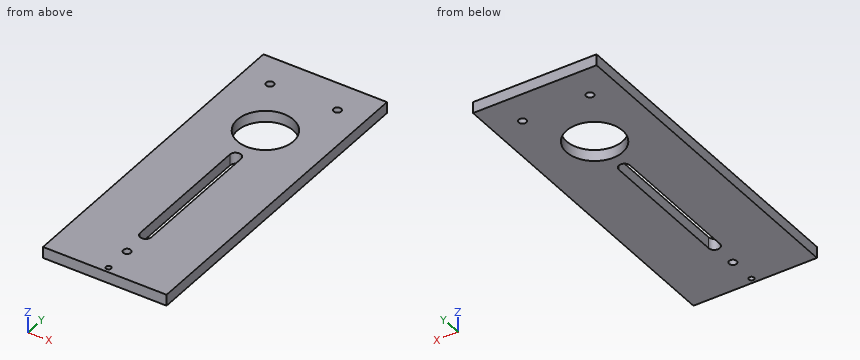
from build123d import *

# Parameters (mm, degrees)
F1_W     = 69.85
F1_H     = 187.2107
F1_R     = 1.4732
F1_R_2   = 2.15265
F1_R_3   = 15.875
F2_DEPTH = 6.35


# Not quite as in the source:
# - a variable given as a bare number and used for a length is read in inches; the dataset says mm whatever the document's units were


with BuildPart() as f2:
    # F1 (on Top) → F2 (new body)
    with BuildSketch(Plane.XY):
        Rectangle(F1_W, F1_H)
        with Locations((0, -90.43035)):
            Circle(F1_R, mode=Mode.SUBTRACT)
        with Locations((0, -74.66965)):
            Circle(F1_R_2, mode=Mode.SUBTRACT)
        with BuildLine():
            ThreePointArc((-3.175, 17.40535), (0, 20.58035), (3.175, 17.40535))
            Line((3.175, 17.40535), (3.175, -58.79465))
            ThreePointArc((3.175, -58.79465), (0, -61.96965), (-3.175, -58.79465))
            Line((-3.175, -58.79465), (-3.175, 17.40535))
        make_face(mode=Mode.SUBTRACT)
        with Locations((-19.05, 75.31735)):
            Circle(F1_R_2, mode=Mode.SUBTRACT)
        with Locations((0, 42.80535)):
            Circle(F1_R_3, mode=Mode.SUBTRACT)
        with Locations((19.05, 75.31735)):
            Circle(F1_R_2, mode=Mode.SUBTRACT)
    extrude(amount=F2_DEPTH)


solid = f2.part
Geometry: final body of the model. Coordinates: model frame, mm. Coordinates: 2 decimals unless noted, no trailing zeros. Loops run counter-clockwise (first coordinate to the right, second up) from the corner with the lowest first, then second, coordinate; pieces in that order, holes last. Notation, with made-up numbers: (45, 17.5) - (77, 17.5) arc R13 cw to (77, 28.5) - close; hole circle Ø8 at (-21, -25.5). An arc over 180 degrees is marked (long way). Put each result on its own line as item: value. Start each with the question number.
Q1. Cut plane A-A, the plane x = -19.05. Return loops of the section in (y, z).
Q2. Line query: line 1 (Y direction, x = 0, z = 2.25); line 2 (X direction, y = 7, z = 4.25) (3 decimals); line 3 (X direction, y = 74, z = 5.5) (1 decimal). Output: solid intervals per line, ascending.
Q3. Pin query (flat end, axial travel): pin 1 Ø1.8 at (x, y) = (0, -90.43) entering from -Z. Return the tip coordinate at first contact, or that it passes through.
Q4. Cut plane B-B, the plane y = -24.5. Return loops of the section in (x, z) (3 decimals).
Q5. Cut plane C-C, the plane z = 4. Return loops of the section in (x, y) (3 decimals), and give its area (3 significant figures).
Filled sheet:
1. outline: (-93.61, 0) - (73.16, 0) - (73.16, 6.35) - (-93.61, 6.35) - close; (77.47, 0) - (93.61, 0) - (93.61, 6.35) - (77.47, 6.35) - close
2. line 1: -93.61 to -91.9, -88.96 to -76.82, -72.52 to -61.97, 20.58 to 26.93, 58.68 to 93.61
2. line 2: -34.925 to -3.175, 3.175 to 34.925
2. line 3: -34.9 to -20.8, -17.3 to 17.3, 20.8 to 34.9
3. pin 1: through
4. outline: (-34.925, 0) - (-3.175, 0) - (-3.175, 6.35) - (-34.925, 6.35) - close; (3.175, 0) - (34.925, 0) - (34.925, 6.35) - (3.175, 6.35) - close
5. outline: (-34.925, -93.605) - (34.925, -93.605) - (34.925, 93.605) - (-34.925, 93.605) - close; hole circle Ø4.305 at (-19.05, 75.317); hole circle Ø31.75 at (0, 42.805); hole (-3.175, -58.795) arc R3.175 ccw to (3.175, -58.795) - (3.175, 17.405) arc R3.175 ccw to (-3.175, 17.405) - close; hole circle Ø4.305 at (0, -74.67); hole circle Ø2.946 at (0, -90.43); hole circle Ø4.305 at (19.05, 75.317)
5. area: 11,700 mm²
